```python
from build123d import *

# Parameters (mm, degrees)
SKETCH_1_W               = 80
SKETCH_1_H               = 70
SKETCH_1_R               = 10
SKETCH_1_R_2             = 1.5
EXTRUDE_1_DEPTH          = 5
EXTRUDE_2_DEPTH          = 55
CUT_EXTRUDE_1_DEPTH      = 60
CUT_EXTRUDE_1_DEPTH_BACK = 60
SKETCH_3_R               = 12
SKETCH_3_R_2             = 1.5
FILLET_3_R               = 1.6
SKETCH_4_R               = 1.5
CUT_EXTRUDE_2_DEPTH      = 10
SKETCH_5_W               = 80
SKETCH_5_H               = 6
CUT_EXTRUDE_3_DEPTH      = 10
FILLET_4_R               = 10
CUT_EXTRUDE_4_DEPTH      = 10
FILLET_5_R               = 5


with BuildPart() as part:
    # 草图1 → 凸台-拉伸1 (new body)
    with BuildSketch(Plane(origin=(0, 0, 0), x_dir=(1, 0, 0), z_dir=(0, 1, 0))):
        Rectangle(SKETCH_1_W, SKETCH_1_H)
        with Locations(Location((0, 0, 0), (0, 0, 270))):
            Circle(SKETCH_1_R, mode=Mode.SUBTRACT)
        with Locations(Location((23, 16, 0), (0, 0, 270))):
            Circle(SKETCH_1_R_2, mode=Mode.SUBTRACT)
        with Locations(Location((23, -6, 0), (0, 0, 90))):
            Circle(SKETCH_1_R_2, mode=Mode.SUBTRACT)
        with Locations(Location((-23, -6, 0), (0, 0, 270))):
            Circle(SKETCH_1_R_2, mode=Mode.SUBTRACT)
        with Locations(Location((-23, 16, 0), (0, 0, 90))):
            Circle(SKETCH_1_R_2, mode=Mode.SUBTRACT)
    extrude(amount=EXTRUDE_1_DEPTH)

    # 草图2 → 凸台-拉伸2 (add)
    with BuildSketch(Plane(origin=(0, 5, 0), x_dir=(1, 0, 0), z_dir=(0, 1, 0))):
        Polygon((-25, -9), (25, -9), (25, -20), (40, -20), (40, -25), (20.5, -25), (20.5, -13), (-20.5, -13), (-20.5, -25), (-40, -25), (-40, -20), (-25, -20), align=None)
    extrude(amount=EXTRUDE_2_DEPTH)

    # 草图3 → 切除-拉伸1 (cut, two sides: drawn at the far end of the back side and taken through both)
    with BuildSketch(Plane.XY.offset(13).offset(-CUT_EXTRUDE_1_DEPTH_BACK)):
        with Locations((0, 26.15)):
            Circle(SKETCH_3_R)
        with Locations((15.5, 41.65)):
            Circle(SKETCH_3_R_2)
        with Locations((15.5, 10.65)):
            Circle(SKETCH_3_R_2)
        with Locations((-15.5, 10.65)):
            Circle(SKETCH_3_R_2)
        with Locations((-15.5, 41.65)):
            Circle(SKETCH_3_R_2)
        with Locations((-30, 13)):
            Circle(SKETCH_3_R_2)
        with Locations((-30, 33)):
            Circle(SKETCH_3_R_2)
        with Locations((-30, 53)):
            Circle(SKETCH_3_R_2)
        with Locations((30, 53)):
            Circle(SKETCH_3_R_2)
        with Locations((30, 33)):
            Circle(SKETCH_3_R_2)
        with Locations((30, 13)):
            Circle(SKETCH_3_R_2)
    extrude(amount=CUT_EXTRUDE_1_DEPTH + CUT_EXTRUDE_1_DEPTH_BACK, mode=Mode.SUBTRACT)

    # 圆角3
    fillet_3_edges = [part.edges().sort_by_distance(p)[0] for p in [
        (25, 32.5, 20),
        (25, 32.5, 9),
        (-25, 32.5, 9),
        (-25, 32.5, 20),
        (-20.5, 32.5, 25),
        (-20.5, 32.5, 13),
        (20.5, 32.5, 13),
        (20.5, 32.5, 25),
    ]]
    fillet(fillet_3_edges, radius=FILLET_3_R)

    # 草图4 → 切除-拉伸2 (cut)
    with BuildSketch(Plane(origin=(0, 5, 0), x_dir=(1, 0, 0), z_dir=(0, 1, 0))):
        with Locations(Location((30, 14, 0), (0, 0, 270))):
            Circle(SKETCH_4_R)
        with Locations(Location((30, -6, 0), (0, 0, 270))):
            Circle(SKETCH_4_R)
        with Locations(Location((-30, -6, 0), (0, 0, 90))):
            Circle(SKETCH_4_R)
        with Locations(Location((-30, 14, 0), (0, 0, 90))):
            Circle(SKETCH_4_R)
    extrude(amount=-CUT_EXTRUDE_2_DEPTH, mode=Mode.SUBTRACT)

    # 草图5 → 切除-拉伸3 (cut)
    with BuildSketch(Plane(origin=(0, 5, 0), x_dir=(1, 0, 0), z_dir=(0, 1, 0))):
        with Locations((0, 32)):
            Rectangle(SKETCH_5_W, SKETCH_5_H)
    extrude(amount=-CUT_EXTRUDE_3_DEPTH, mode=Mode.SUBTRACT)

    # 圆角4
    fillet_4_edges = [part.edges().sort_by_distance(p)[0] for p in [
        (-40, 2.5, -29),
        (40, 2.5, -29),
        (40, 2.5, 35),
        (-40, 2.5, 35),
    ]]
    fillet(fillet_4_edges, radius=FILLET_4_R)

    # 草图6 → 切除-拉伸4 (cut)
    with BuildSketch(Plane.XY.offset(13)):
        with BuildLine():
            Line((18.9, 60), (-18.9, 60))
            add(Edge.make_bspline(
                [(-18.9, 60), (-11.034609478, 52.202200448), (0, 52)],
                knots=[0, 0, 0, 1, 1, 1], degree=2))
            add(Edge.make_bspline(
                [(18.9, 60), (11.034609478, 52.202200448), (0, 52)],
                knots=[0, 0, 0, 1, 1, 1], degree=2))
        make_face()
    extrude(amount=-CUT_EXTRUDE_4_DEPTH, mode=Mode.SUBTRACT)

    # 圆角5
    fillet_5_edges = [part.edges().sort_by_distance(p)[0] for p in [
        (-40, 60, 22.5),
        (40, 60, 22.5),
    ]]
    fillet(fillet_5_edges, radius=FILLET_5_R)


solid = part.part
```
For this review, take the finished solid that the model builds, in its own axes (mm). A direction names the side the tool comes from. Round coordinates to 2 decimals unless told otherwise and drop trailing zeros. Write each loop counter-clockwise with the first axis right and the second up, starting at its lowest first coordinate (ties: lowest second). Pieces come first, ordered by that corner, then holes. Notation, with made-up numbers: (53, 24) -> (78, 24) arc R19 cw to (78, 42) -> close; hole circle Ø9 at (-33, 28.5). An arc over 180 degrees is marked (long way). One line per question, with ' | ' between items. Start each with the question number.
(1) Add section B-B, the plane z = 6. Write out the cut boundary in (x, y).
(2) Add section A-A, the plane y = 41.65. Write out the cut boundary in (x, z).
(3) For line 1 along X through (y, z) = (13, 21.4); line 2 along Z through (x, y) = (-30, 2.9); line 3 along Y through (x, z) = (0, 11.6), list the stretches that pass through material, from the lowest coordinate up. Write a range as from..to.
(4) Mouldability with a two-part tool opening along X and no side actions: class faces 1 (the face through (-9, 0, 10)), 2 (the face through (28.8, 32.1, 22.5)), 3 (the face through (-40, 15, 21)) as released by +X, released by -X, zero draft, split by the parting line, or undercut.
(5) Tool access review of faces 4 (the face through (31.01, 2.54, 4.89)), 5 (the face through (39, 58, 23)), 6 (the face through (-33, 32, 25)), 7 (the face through (-25, 32, 15)), 8 (the face through (20.5, 32, 19)): name each direction out of +Z, -Z, +X, -X, +Y, -Y from which nothing blocks a thin tool from reaching the whole face with its end or side.
(6) Insertion check: P1, Ø4, axis at x = 21, y = 11, coming from the +Z side; P2, Ø3.5, axis at x = 30, z = -14, coming from the +Y side; P3, Ø16, axis at x = 0, z = 0, coming from the -Y side; P4, Ø4.5, axis at y = 24, z = 17.5, coming from the -X side. Each pin has a flat end and moves straight along its axis. Give the tip position at first contact, or say it passes through.
(7) Add section C-C, the plane y = 33. Give the number of separate pieces and of enclosed holes in the cut face, plus the area to 3 significant figures.
Answer list:
1) outline: (-40, 0) -> (-31.5, 0) -> (-31.5, 5) -> (-40, 5) -> close; (-28.5, 0) -> (-24.5, 0) -> (-24.5, 5) -> (-28.5, 5) -> close; (-21.5, 0) -> (-8, 0) -> (-8, 5) -> (-21.5, 5) -> close; (8, 0) -> (21.5, 0) -> (21.5, 5) -> (8, 5) -> close; (24.5, 0) -> (28.5, 0) -> (28.5, 5) -> (24.5, 5) -> close; (31.5, 0) -> (40, 0) -> (40, 5) -> (31.5, 5) -> close
2) outline: (-40, 20) -> (-26.6, 20) arc R1.6 cw to (-25, 18.4) -> (-25, 10.6) arc R1.6 ccw to (-23.4, 9) -> (-17, 9) -> (-17, 13) -> (-18.9, 13) arc R1.6 cw to (-20.5, 14.6) -> (-20.5, 23.4) arc R1.6 ccw to (-22.1, 25) -> (-40, 25) -> close; (-14, 9) -> (14, 9) -> (14, 13) -> (-14, 13) -> close; (17, 9) -> (23.4, 9) arc R1.6 ccw to (25, 10.6) -> (25, 18.4) arc R1.6 cw to (26.6, 20) -> (40, 20) -> (40, 25) -> (22.1, 25) arc R1.6 ccw to (20.5, 23.4) -> (20.5, 14.6) arc R1.6 cw to (18.9, 13) -> (17, 13) -> close
3) line 1: -40..-31.5, -28.5..-20.5, 20.5..28.5, 31.5..40 | line 2: -29..-15.5, -12.5..4.5, 7.5..35 | line 3: 0..14.15, 38.15..52
4) face 1: zero draft | face 2: undercut | face 3: released by -X
5) face 4: +Y, -Y | face 5: +Z, -Z, +X, +Y | face 6: +Z, +X, -X, +Y | face 7: -Z, -X, +Y | face 8: +Z, +Y
6) P1: z = 25 | P2: y = 5 | P3: through | P4: x = -25.74
7) separate pieces: 4 | enclosed holes: 0 | area: 349 mm²
